```python
from build123d import *

# Parameters (mm, degrees)
F0_R      = 2.25
F1_DEPTH  = 10
F3_DEPTH  = 20
F4_R      = 2.25
F5_DEPTH  = 5
F6_R      = 2.25
F7_DEPTH  = 5
F8_R      = 3.75
F9_DEPTH  = 2
F10_R     = 3.75
F11_DEPTH = 2


with BuildPart() as f1:
    # F0 (on Top) → F1 (new body)
    with BuildSketch(Plane.XY):
        Polygon((20, 20), (0, 20), (0, 0), (20, 0), (40, 20), (60, 20.106066), (60, 40), (20, 40), align=None)
        with Locations((30, 30)):
            Circle(F0_R, mode=Mode.SUBTRACT)
        with Locations((45, 30)):
            Circle(F0_R, mode=Mode.SUBTRACT)
    extrude(amount=F1_DEPTH)

    # F2 (on face) → F3 (join)
    with BuildSketch(Plane.XY.offset(10)):
        Polygon((40, 20), (20, 20), (20, 0), (25, 5), (25, 10), (25, 15), (30, 15), (35, 15), align=None)
    extrude(amount=F3_DEPTH)

    # F4 (on face) → F5 (cut)
    with BuildSketch(Plane(origin=(20, 0, 0), x_dir=(0, -1, 0), z_dir=(-1, 0, 0))):
        with Locations((-7, 20)):
            Circle(F4_R)
    extrude(amount=-F5_DEPTH, mode=Mode.SUBTRACT)

    # F6 (on face) → F7 (cut)
    with BuildSketch(Plane(origin=(0, 20, 0), x_dir=(-1, 0, 0), z_dir=(0, 1, 0))):
        with Locations((-33, 20)):
            Circle(F6_R)
    extrude(amount=-F7_DEPTH, mode=Mode.SUBTRACT)

    # F8 (on face) → F9 (cut)
    with BuildSketch(Plane.XZ.offset(-15)):
        with Locations((33, 20)):
            Circle(F8_R)
    extrude(amount=-F9_DEPTH, mode=Mode.SUBTRACT)

    # F10 (on face) → F11 (cut)
    with BuildSketch(Plane.YZ.offset(25)):
        with Locations((7, 20)):
            Circle(F10_R)
    extrude(amount=-F11_DEPTH, mode=Mode.SUBTRACT)


solid = f1.part
```
Design review of the part built by this model. Coordinates are the model's own, in mm. A direction names the side the tool comes from. Coordinates: 2 decimals unless noted, no trailing zeros. Loops run counter-clockwise (first coordinate to the right, second up) from the corner with the lowest first, then second, coordinate; pieces in that order, holes last. Notation, with made-up numbers: (-7, -31.75) - (51, -31.75) arc R27 cw to (51, 7.25) - close; hole circle Ø11 at (-39, 48). An arc over 180 degrees is marked (long way). Use CSV: the item, a comma, the result in double quotes. Start each with the question number.
1) Consider section A-A on y = 7. Write out the cut boundary in (x, z).
2) The part is to be moulded in two halves that separate along Z. For faces 5 (the flat face through (29, 11, 10)), 6 (the cylindrical face through (23.996, 10.577, 21.126)), 7 (the flat face through (30, 20, 20)), say which applies: +Z half, -Z half, draft (parallel to the pull), parting line (faces both ways), or undercut.
3) Consider section C-C on y = 30. Write out the cut boundary in (x, z).
4) For pin 1 Ø3 at (y, z) = (11, 18) entering from +X; pin 2 Ø10 at (y, z) = (19.5, 16) entering from -X; pin 3 Ø8 at (x, z) = (42.5, 20.5) entering from -Y; pin 4 Ø2.5 at (x, y) = (45, 30) entering from +Z, all flat-tipped, find the tip position at first contact; note any pin that passes through.
5) Tool access review of faces 1 (the flat face through (25, 11, 20)), 2 (the flat face through (10, 20, 5)), 3 (the flat face through (35, 17, 18)), 4 (the flat face through (20, 10, 20)): name each direction out of +Z, -Z, +X, -X, +Y, -Y from which nothing blocks a thin tool from reaching the whole face with its end or side.
6) Consider section D-D on z = 20. Write out the cut boundary in (x, y).
7) Wall thickness on L1, parallel to Z at x = 21.3, y = 7; L2, parallel to Y at x = 30, z = 2; L3, parallel to X at y = 10, z = 13.5: over which ranges is each line inside the solid? List them lowest first. Write a range as from..to.
8) Consider section B-B on x = 30. Write out the cut boundary in (y, z).
Geometry says:
1,outline,"(0, 0) - (27, 0) - (27, 10) - (25, 10) - (25, 16.25) - (23, 16.25) - (23, 17.75) - (20, 17.75) - (20, 10) - (0, 10) - close; (20, 22.25) - (23, 22.25) - (23, 23.75) - (25, 23.75) - (25, 30) - (20, 30) - close"
2,face 5,"+Z half"
2,face 6,"undercut"
2,face 7,"draft"
3,outline,"(20, 0) - (27.75, 0) - (27.75, 10) - (20, 10) - close; (32.25, 0) - (42.75, 0) - (42.75, 10) - (32.25, 10) - close; (47.25, 0) - (60, 0) - (60, 10) - (47.25, 10) - close"
4,pin 1,"x = 25"
4,pin 2,"x = 20"
4,pin 3,"y = 18.5"
4,pin 4,"through"
5,face 1,"+Z, +X, -Y"
5,face 2,"+Z, -Z, -X, +Y"
5,face 3,"-Y"
5,face 4,"+Z, -X, +Y, -Y"
6,outline,"(20, 0) - (23.25, 3.25) - (23, 3.25) - (23, 4.75) - (20, 4.75) - close; (20, 9.25) - (23, 9.25) - (23, 10.75) - (25, 10.75) - (25, 15) - (29.25, 15) - (29.25, 17) - (30.75, 17) - (30.75, 20) - (20, 20) - close; (35.25, 17) - (36.75, 17) - (36.75, 16.75) - (40, 20) - (35.25, 20) - close"
7,L1,"0..17.75, 22.25..30"
7,L2,"10..27.75, 32.25..40"
7,L3,"20..25"
8,outline,"(10, 0) - (27.75, 0) - (27.75, 10) - (20, 10) - (20, 30) - (15, 30) - (15, 22.25) - (17, 22.25) - (17, 17.75) - (15, 17.75) - (15, 10) - (10, 10) - close; (32.25, 0) - (40, 0) - (40, 10) - (32.25, 10) - close"
